```python
from build123d import *

# Parameters (mm, degrees)
F1_DEPTH = 4.5
F2_SIZE  = 1.19999
F3_R     = 1.05
F4_DEPTH = 25


# Not quite as in the source:
# - a fillet or chamfer is up to 0.001 mm smaller than in the source, because OpenCascade refuses the exact size


with BuildPart() as f1:
    # F0 (on Front) → F1 (new body)
    with BuildSketch(Plane.XZ):
        Polygon((-3.8, 1.2), (-3.8, 0), (-2.6, 0), (2.6, 0), (3.8, 0), (3.8, 1.2), (2.6, 3.4), (2.6, 4.6), (3.8, 4.6), (3.8, 5.8), (2.6, 8), (2.6, 9.2), (3.8, 9.2), (3.8, 10.4), (2.6, 12.6), (2.6, 13.8), (3.8, 13.8), (3.8, 15), (2.6, 17.2), (2.6, 18.4), (3.8, 18.4), (3.8, 19.6), (2.6, 21.8), (2.6, 23), (3.8, 23), (3.8, 24.2), (2.6, 26.4), (2.6, 27.6), (3.8, 27.6), (3.8, 28.8), (2.6, 31), (2.6, 32.2), (3.8, 32.2), (3.8, 33.4), (2.6, 35.6), (2.6, 36.8), (3.8, 36.8), (3.8, 38), (2.6, 40.2), (2.6, 41.4), (3.8, 41.4), (3.8, 42.6), (2.6, 44.8), (2.6, 46), (3.8, 46), (3.8, 47.2), (2.6, 49.4), (2.6, 50.6), (3.8, 50.6), (3.8, 51.8), (2.6, 54), (2.6, 55.2), (3.8, 55.2), (3.8, 56.4), (2.6, 58.6), (2.6, 59.8), (3.8, 59.8), (3.8, 61), (2.6, 63.2), (2.6, 64.4), (3.8, 64.4), (3.8, 65.6), (2.6, 67.8), (2.6, 69), (3.8, 69), (3.8, 70.2), (2.6, 72.4), (2.6, 73.6), (3.8, 73.6), (3.8, 74.8), (2.6, 77), (2.6, 78.2), (3.8, 78.2), (3.8, 79.4), (2.6, 81.6), (2.6, 82.8), (3.8, 82.8), (3.8, 84), (2.6, 86.2), (2.6, 87.4), (3.8, 87.4), (3.8, 88.6), (2.6, 90.8), (2.6, 92), (-2.6, 92), (-2.6, 90.8), (-3.8, 88.6), (-3.8, 87.4), (-2.6, 87.4), (-2.6, 86.2), (-3.8, 84), (-3.8, 82.8), (-2.6, 82.8), (-2.6, 81.6), (-3.8, 79.4), (-3.8, 78.2), (-2.6, 78.2), (-2.6, 77), (-3.8, 74.8), (-3.8, 73.6), (-2.6, 73.6), (-2.6, 72.4), (-3.8, 70.2), (-3.8, 69), (-2.6, 69), (-2.6, 67.8), (-3.8, 65.6), (-3.8, 64.4), (-2.6, 64.4), (-2.6, 63.2), (-3.8, 61), (-3.8, 59.8), (-2.6, 59.8), (-2.6, 58.6), (-3.8, 56.4), (-3.8, 55.2), (-2.6, 55.2), (-2.6, 54), (-3.8, 51.8), (-3.8, 50.6), (-2.6, 50.6), (-2.6, 49.4), (-3.8, 47.2), (-3.8, 46), (-2.6, 46), (-2.6, 44.8), (-3.8, 42.6), (-3.8, 41.4), (-2.6, 41.4), (-2.6, 40.2), (-3.8, 38), (-3.8, 36.8), (-2.6, 36.8), (-2.6, 35.6), (-3.8, 33.4), (-3.8, 32.2), (-2.6, 32.2), (-2.6, 31), (-3.8, 28.8), (-3.8, 27.6), (-2.6, 27.6), (-2.6, 26.4), (-3.8, 24.2), (-3.8, 23), (-2.6, 23), (-2.6, 21.8), (-3.8, 19.6), (-3.8, 18.4), (-2.6, 18.4), (-2.6, 17.2), (-3.8, 15), (-3.8, 13.8), (-2.6, 13.8), (-2.6, 12.6), (-3.8, 10.4), (-3.8, 9.2), (-2.6, 9.2), (-2.6, 8), (-3.8, 5.8), (-3.8, 4.6), (-2.6, 4.6), (-2.6, 3.4), align=None)
    extrude(amount=F1_DEPTH)

    # F2 (size 1.2 in the source; OpenCascade refuses exactly that, so slightly less here)
    f2_edges = [f1.edges().sort_by_distance(p)[0] for p in [
        (2.6, -2.25, 92),
        (-2.6, -2.25, 92),
    ]]
    chamfer(f2_edges, length=F2_SIZE)

    # F3 (on face) → F4 (cut)
    with BuildSketch(Plane.XZ.offset(4.5)):
        with Locations((0, 90)):
            Circle(F3_R)
    extrude(amount=-F4_DEPTH, mode=Mode.SUBTRACT)


solid = f1.part
```
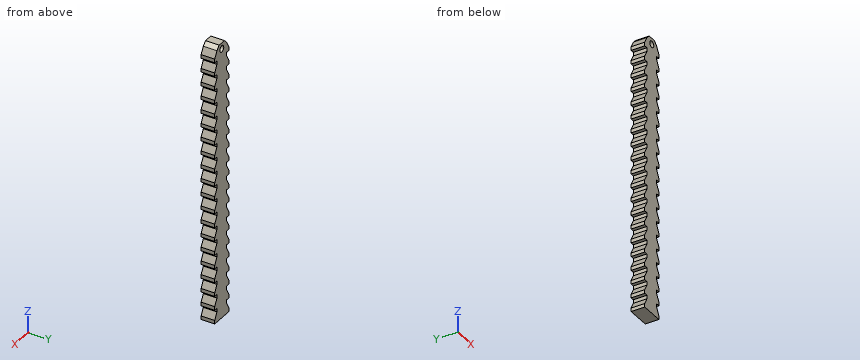
Verification items for the finished model (mm, model axes). Round coordinates to 2 decimals unless told otherwise and drop trailing zeros. Order: outer loops, then holes, each group sorted by start corner. A loop starts at its lowest first (then second) coordinate and runs counter-clockwise, first axis right, second up. Notation, with made-up numbers: (5.25, 24.25) - (59.25, 24.25) arc R8 ccw to (59.25, 31.25) - close; hole circle Ø3 at (2, 42.25). An arc over 180 degrees is marked (long way). Use CSV: the item, a comma, the result in double quotes.
(1) Gauge pin test, flat ends, axial feed: pin 1 Ø0.6 at (y, z) = (-2.5, 54.5) entering from -X; pin 2 Ø2 at (x, y) = (3, -3.5) entering from +Z. Record the tip position at first contact, or that the pin passes through.
Entries:
pin 1,"x = -2.6"
pin 2,"z = 91.4"
(2) Section check B-B on z = 90. Record the boundary of the cut face in (x, y).
Entries:
outline,"(-3.04, -4.5) - (-1.05, -4.5) - (-1.05, 0) - (-3.04, 0) - close; (1.05, -4.5) - (3.04, -4.5) - (3.04, 0) - (1.05, 0) - close"
(3) Section check A-A on x = 0. Record the boundary of the cut face in (y, z).
Entries:
outline,"(-4.5, 0) - (0, 0) - (0, 88.95) - (-4.5, 88.95) - close; (-4.5, 91.05) - (0, 91.05) - (0, 92) - (-4.5, 92) - close"
(4) Thickness scan on probe 1 along Z at (x, y) = (0, -3.2); probe 2 along X at (y, z) = (-2.05, 90); probe 3 along Z at (x, y) = (0.75, -3.6). Record the ranges inside material, lowest first. Write a range as from..to.
Entries:
probe 1,"0..88.95, 91.05..92"
probe 2,"-3.04..-1.05, 1.05..3.04"
probe 3,"0..89.27, 90.73..92"
